Autodesk Inventor part; units mm, degrees
ref_plane "YZ Plane" through (0, 0, 0) normal (1, 0, 0) x (0, 1, 0)
ref_plane "XZ Plane" through (0, 0, 0) normal (0, 1, 0) x (-1, 0, 0)
ref_plane "XY Plane" through (0, 0, 0) normal (0, 0, 1) x (1, 0, 0)
sketch "Sketch1" plane through (0, 0, 0) normal (1, 0, 0) x (0, 1, 0)
  circle A0 centre (0, 0) radius 11.2253
extrude "Extrusion1" add sketch "Sketch1" along normal blind 12.7
sketch "Sketch2" plane through (0, 0, 0) normal (-1, 0, 0) x (0, 0, 1)
  line L0 (-4.7625, 0) -> (-2.3813, 4.1244)
  line L1 (-2.3813, 4.1244) -> (2.3812, 4.1244)
  line L2 (2.3812, 4.1244) -> (4.7625, 0)
  line L3 (4.7625, 0) -> (2.3813, -4.1244)
  line L4 (2.3813, -4.1244) -> (-2.3812, -4.1244)
  line L5 (-2.3812, -4.1244) -> (-4.7625, 0)
  circle A0 centre (0, 0) radius 1.5875
  point P0 (1.6165, 3.316)
extrude "Extrusion2" add sketch "Sketch2" along normal blind 2.54
sketch "Sketch3" plane through (-2.54, 0, 0) normal (-1, 0, 0) x (0, 0, 1)
  circle A0 centre (0, 0) radius 1.143
  dimension "d4" = 2.286
extrude "Extrusion3" add sketch "Sketch3" along normal blind 13.6525 and the other way blind 8.4201
sketch "Sketch4" plane through (12.7, 0, 0) normal (1, 0, 0) x (0, 0, -1)
  circle A0 centre (0, 0) radius 7.0995
extrude "Extrusion4" add sketch "Sketch4" along normal blind 11.1125
properties part number "DC MOTOR NEW"
Source: CAD feature listing. Evaluate the final solid. Frame: model axes, mm. A direction names the side the tool comes from. Round coordinates to 2 decimals unless told otherwise and drop trailing zeros. Write each loop counter-clockwise with the first axis right and the second up, starting at its lowest first coordinate (ties: lowest second). Pieces come first, ordered by that corner, then holes. Notation, with made-up numbers: M 78.5,11.25 L 122.5,11.25 A28 ccw 122.5,31.25 Z; hole C 73,68.5 d4. An arc over 180 degrees is marked long. Answer as a JSON object with one key per item and string values. Group by question number.
(1) Ray query, line 1 (Y direction, x = -0.65, z = 0); line 2 (X direction, y = -3.25, z = 6.5); line 3 (X direction, y = 4, z = 2.5). Return the intervals inside material, ascending. Write a range as [from, to].
(2) Section query D-D on z = 6.25. Output: boundary loops of the cut face in (x, y).
(3) Section query A-A on z = 0. Output: boundary loops of the cut face in (x, y).
(4) Section query B-B on y = -3. Output: boundary loops of the cut face in (x, z), then the cut area to 3 significant figures.
(5) Mould query, pull axis Z, two halves, no side actions, for faces 6 (the flat face through (-1.252, 2.091, 3.555)), 7 (the cylindrical face through (-1.25, 1.55, -0.34)), 8 (the flat face through (0, 0, -5)), 9 (the flat face through (0, 1, -1)). Classes: +Z half, -Z half, draft (parallel to the pull), parting line (faces both ways), or undercut.
(6) First-contact query: pin 1 (4 mm diameter, centred on y = -7.5, z = 1, fed in from -X); pin 2 (2 mm diameter, centred on x = 9.5, z = 2.5, fed in from -Y); pin 3 (3 mm diameter, centred on x = -1, z = -0.5, fed in from -Y); pin 4 (1.5 mm diameter, centred on x = 15, z = 2.5, fed in from -Y). Flat tips, straight axial feed; report the tip coordinate or a pass-through.
(7) Reachability of faces 1 (the flat face through (-1.25, -2.03, 3.59)), 2 (the cylindrical face through (-8.21, -1.116, -0.248)), 3 (the flat face through (-1.252, -2.091, -3.555)), 4 (the flat face through (12.7, 7.3, 0.2)), 5 (the flat face through (-1.25, 2.03, -3.59)) from +Z, -Z, +X, -X, +Y, -Y: full face, straight path, thin tool, end or side. Return the list, or none.
(8) Section query C-C on x = 7.5. Output: boundary loops of the cut face in (y, z), then the cut area to 3 significant figures.
Computed values:
{
 "1": {"line 1": "[-4.12, -1.59], [-1.14, 1.14], [1.59, 4.12]", "line 2": "[0, 12.7]", "line 3": "[0, 23.81]"},
 "2": {"outline": "M 0,-9.32 L 12.7,-9.32 L 12.7,-3.37 L 23.81,-3.37 L 23.81,3.37 L 12.7,3.37 L 12.7,9.32 L 0,9.32 Z"},
 "3": {"outline": "M -16.19,-1.14 L 0,-1.14 L 0,-1.59 L -2.54,-1.59 L -2.54,-4.12 L 0,-4.12 L 0,-11.23 L 12.7,-11.23 L 12.7,-7.1 L 23.81,-7.1 L 23.81,7.1 L 12.7,7.1 L 12.7,11.23 L 0,11.23 L 0,4.12 L -2.54,4.12 L -2.54,1.59 L 0,1.59 L 0,1.14 L -16.19,1.14 Z"},
 "4": {"outline": "M -2.54,-3.03 L 0,-3.03 L 0,-10.82 L 12.7,-10.82 L 12.7,-6.43 L 23.81,-6.43 L 23.81,6.43 L 12.7,6.43 L 12.7,10.82 L 0,10.82 L 0,3.03 L -2.54,3.03 Z", "area": "433 mm^2"},
 "5": {"face 6": "+Z half", "face 7": "undercut", "face 8": "draft", "face 9": "undercut"},
 "6": {"pin 1": "x = 0", "pin 2": "y = -11.12", "pin 3": "y = -11.23", "pin 4": "y = -6.88"},
 "7": {"face 1": "+Z, -X, -Y", "face 2": "-X", "face 3": "-Z, -X, -Y", "face 4": "+X", "face 5": "-Z, -X, +Y"},
 "8": {"outline": "C 0,0 d22.45", "area": "396 mm^2"}
}
